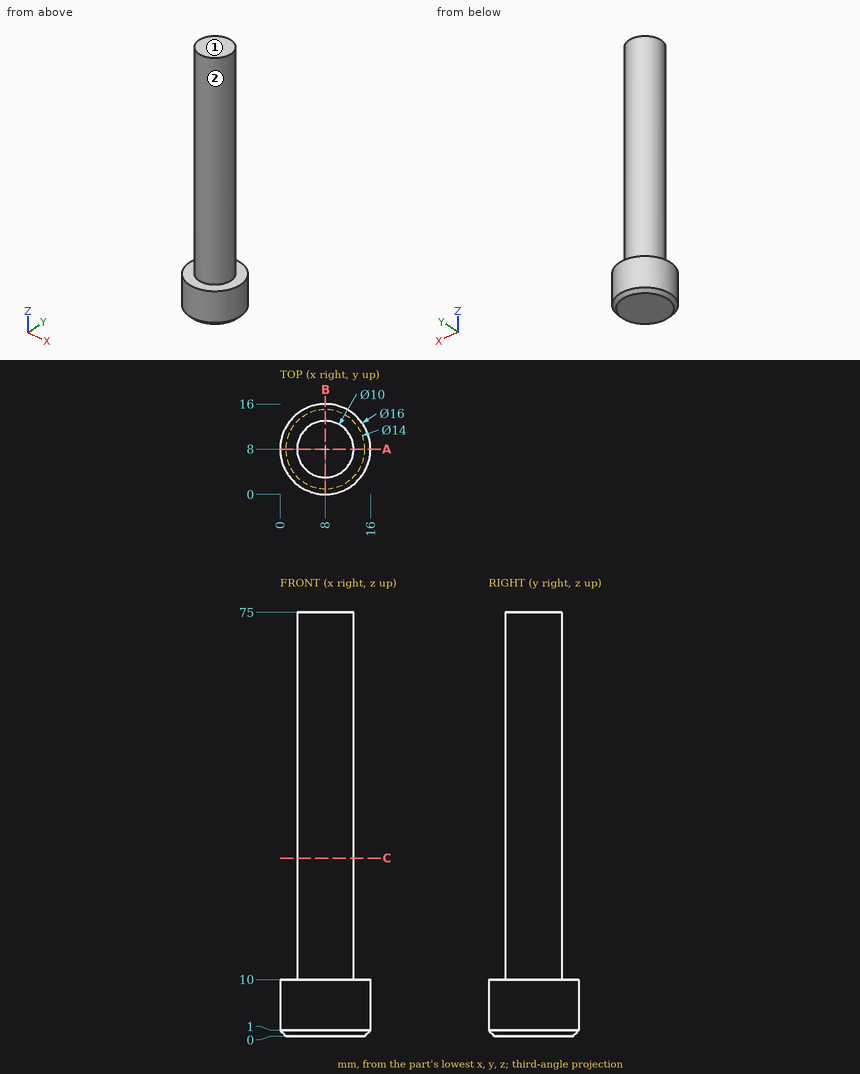
Drawing for the job (mm, zero at the part's lowest x, y, z). A direction names the side the tool comes from. Round coordinates to 2 decimals unless told otherwise and drop trailing zeros. Write each loop counter-clockwise with the first axis right and the second up, starting at its lowest first coordinate (ties: lowest second). Pieces come first, ordered by that corner, then holes. Notation, with made-up numbers: M -28,16.5 L -20,16.5 A21 ccw -20,37.5 Z; hole C 23,25.25 d4. An arc over 180 degrees is marked long. One line per question, with ' | ' between items.
1. Cut at A-A on y = 8. Write the cut outline in (x, z), and give its area (3 significant figures).
Working result:
outline: M 0,1 L 1,0 L 15,0 L 16,1 L 16,10 L 13,10 L 13,75 L 3,75 L 3,10 L 0,10 Z | area: 809 mm2
2. Cut at C-C on z = 31.5. Write the cut outline in (x, y).
Working result:
outline: C 8,8 d10
3. Which spindle directions (+Z, -Z, +X, -X, +Y, -Y) get a long thin tool onto all of the face, cutting with end or side? Do the marked faces 1 and 2. Say none if no direction does.
Working result:
face 1: +Z, +X, -X, +Y, -Y | face 2: +Z
4. Probe L1, parallel to X at y = 7.5, z = 8; L2, parallel to Z at x = 3.75, y = 3.5; L3, parallel to Y at x = 8.25, z = 41.5. List the from-to ranges inside material, lowest first. Write a range as from..to.
Working result:
L1: 0.02..15.98 | L2: 0..10 | L3: 3.01..12.99
5. Pin check, flat tips, straight feed: pin 1 Ø1 at (x, z) = (13, 63) entering from -Y; pin 2 Ø4 at (x, z) = (11, 33.5) entering from +Y; pin 3 Ø8 at (x, z) = (3.5, 32.5) entering from -Y. Stop position of each tip, or through.
Working result:
pin 1: y = 5.82 | pin 2: y = 12.9 | pin 3: y = 3.03
